```python
from build123d import *

# Parameters (mm, degrees)
F0_R      = 3.25
F1_DEPTH  = 2.5
F2_R      = 4
F2_R_2    = 3.25
F3_DEPTH  = 5
F4_R      = 6
F4_R_2    = 4
F5_DEPTH  = 5
F7_DEPTH  = 3
F8_R      = 5.5
F9_DEPTH  = 3
F10_R     = 5
F11_DEPTH = 1.25
F12_R     = 5.125
F12_R_2   = 5
F13_DEPTH = 1.5
F14_W     = 7.2478445072
F14_H     = 7.2478445072
F15_DEPTH = 7
F16_R     = 2.75
F17_DEPTH = 5
F18_R     = 0.25
F19_DEPTH = 4.5


with BuildPart() as f1:
    # F0 (on Top) → F1 (new body)
    with BuildSketch(Plane.XY):
        Circle(F0_R)
    extrude(amount=-F1_DEPTH)

    # F2 (on face) → F3 (join)
    with BuildSketch(Plane(origin=(0, 0, -2.5), x_dir=(1, 0, 0), z_dir=(0, 0, -1))):
        Circle(F2_R)
        Circle(F2_R_2, mode=Mode.SUBTRACT)
        Circle(F2_R_2)
    extrude(amount=F3_DEPTH)

    # F4 (on face) → F5 (join)
    with BuildSketch(Plane(origin=(0, 0, -7.5), x_dir=(1, 0, 0), z_dir=(0, 0, -1))):
        Circle(F4_R)
        Circle(F4_R_2, mode=Mode.SUBTRACT)
        Circle(F4_R_2)
    extrude(amount=F5_DEPTH)

    # F6 (on face) → F7 (join)
    with BuildSketch(Plane(origin=(0, 0, -12.5), x_dir=(1, 0, 0), z_dir=(0, 0, -1))):
        Polygon((4.8541019662, -3.5267115138), (6, 0), (4.8541019662, 3.5267115138), (1.8541019662, 5.7063390978), (-1.8541019662, 5.7063390978), (-4.8541019662, 3.5267115138), (-6, 0), (-4.8541019662, -3.5267115138), (-1.8541019662, -5.7063390978), (1.8541019662, -5.7063390978), align=None)
    extrude(amount=F7_DEPTH)

    # F8 (on face) → F9 (join)
    with BuildSketch(Plane(origin=(0, 0, -15.5), x_dir=(1, 0, 0), z_dir=(0, 0, -1))):
        Circle(F8_R)
    extrude(amount=F9_DEPTH)

    # F10 (on face) → F11 (join)
    with BuildSketch(Plane(origin=(0, 0, -18.5), x_dir=(1, 0, 0), z_dir=(0, 0, -1))):
        Circle(F10_R)
    extrude(amount=F11_DEPTH)

    # F12 (on face) → F13 (join)
    with BuildSketch(Plane(origin=(0, 0, -19.75), x_dir=(1, 0, 0), z_dir=(0, 0, -1))):
        Circle(F12_R)
        Circle(F12_R_2, mode=Mode.SUBTRACT)
        Circle(F12_R_2)
    extrude(amount=F13_DEPTH)

    # F14 (on face) → F15 (join)
    with BuildSketch(Plane(origin=(0, 0, -21.25), x_dir=(1, 0, 0), z_dir=(0, 0, -1))):
        Rectangle(F14_W, F14_H)
    extrude(amount=F15_DEPTH)

    # F16 (on face) → F17 (cut)
    with BuildSketch(Plane.XY):
        Circle(F16_R)
    extrude(amount=-F17_DEPTH, mode=Mode.SUBTRACT)

    # F18 (on face) → F19 (join)
    with BuildSketch(Plane.XY.offset(-5)):
        with Locations((-1.25, -1.25)):
            Circle(F18_R)
        with Locations((1.25, -1.5)):
            Circle(F18_R)
        with Locations((1.25, 1.5)):
            Circle(F18_R)
        with Locations((-1.25, 1.25)):
            Circle(F18_R)
    extrude(amount=F19_DEPTH)


solid = f1.part
```
Work out the finished part from the listing and answer in its coordinate system (mm). A direction names the side the tool comes from. Coordinates: 2 decimals unless noted, no trailing zeros. Loops run counter-clockwise (first coordinate to the right, second up) from the corner with the lowest first, then second, coordinate; pieces in that order, holes last.
1) Section A-A (z = -23.5) is taken. Give the vertices of the cut face in (x, y), plus the area to 3 significant figures.
Results:
outline: (-3.62, -3.62) - (3.62, -3.62) - (3.62, 3.62) - (-3.62, 3.62) - close
area: 52.5 mm2
2) Section B-B (z = -8) is taken. Give the vertices of the cut face in (x, y), plus the area to 3 significant figures.
Results:
outline: circle Ø12 at (0, 0)
area: 113 mm2
3) Flat-ended cylindrical pins translate along their axes: pin 1 (5 mm diameter, centred on x = -0.5, z = -4.5, fed in from -Y); pin 2 (3.5 mm diameter, centred on y = -1.5, z = -25, fed in from -X); pin 3 (1 mm diameter, centred on x = 1.5, y = -0.5, fed in from +Z). Find the tip coordinate at first contact, or state that the pin passes through.
Results:
pin 1: stops at y = -4
pin 2: stops at x = -3.62
pin 3: stops at z = -5
4) For faces 1 (the flat face through (-1.42, 3.92, -7.5)), 2 (the flat face through (5.435, -1.739, -13.979)), 3 (the flat face through (0, 4, -21.25)), 4 (the flat face through (-3.624, 0, -25)), determine the directions among +Z, -Z, +X, -X, +Y, -Y from which every point of the face is accessible in a straight line to the end or side of a thin tool.
Results:
face 1: +Z
face 2: -Z, +X, -Y
face 3: -Z, +X, -X, +Y
face 4: -Z, -X, +Y, -Y
5) Section C-C (z = -16.5) is taken. Give the vertices of the cut face in (x, y), plus the area to 3 significant figures.
Results:
outline: circle Ø11 at (0, 0)
area: 95.0 mm2
6) Consider probe 1 along Y at (x, z) = (0, -3.1); probe 2 along Y at (x, z) = (0, -2.2); probe 3 along Z at (x, y) = (-0.5, 1). Determine where each line is inside the solid, lowest interval first.
Results:
probe 1: y = -4 to -2.75, 2.75 to 4
probe 2: y = -3.25 to -2.75, 2.75 to 3.25
probe 3: z = -28.25 to -5
